from build123d import *

# Parameters (mm, degrees)
SKETCH1_R           = 25
BOSS_EXTRUDE1_DEPTH = 40
SKETCH2_R           = 60
BOSS_EXTRUDE2_DEPTH = 50
CHAMFER1_SIZE       = 7.5
CUT_EXTRUDE1_DEPTH  = 3


with BuildPart() as part:
    # Sketch1 → Boss-Extrude1 (new body)
    with BuildSketch(Plane(origin=(0, 0, 0), x_dir=(1, 0, 0), z_dir=(0, 1, 0))):
        with Locations(Location((0, 0, 0), (0, 0, 270))):
            Circle(SKETCH1_R)
    extrude(amount=BOSS_EXTRUDE1_DEPTH)

    # Sketch2 → Boss-Extrude2 (add)
    with BuildSketch(Plane(origin=(0, 40, 0), x_dir=(1, 0, 0), z_dir=(0, 1, 0))):
        with Locations(Location((0, 0, 0), (0, 0, 270))):
            Circle(SKETCH2_R)
    extrude(amount=BOSS_EXTRUDE2_DEPTH)

    # Chamfer1
    chamfer1_edges = [part.edges().sort_by_distance(p)[0] for p in [
        (0, 90, -60),
    ]]
    chamfer(chamfer1_edges, length=CHAMFER1_SIZE)

    # Sketch3 → Cut-Extrude1 (cut)
    with BuildSketch(Plane(origin=(0, 90, 0), x_dir=(1, 0, 0), z_dir=(0, 1, 0))):
        with BuildLine():
            Line((-3, 1.732050808), (-53.461524227, -27.401923789))
            ThreePointArc((-53.461524227, -27.401923789), (-54.559600438, -31.5), (-50.461524227, -32.598076211))
            Line((-50.461524227, -32.598076211), (0, -3.464101615))
            Line((0, -3.464101615), (50.461524227, -32.598076211))
            ThreePointArc((50.461524227, -32.598076211), (54.559600438, -31.5), (53.461524227, -27.401923789))
            Line((53.461524227, -27.401923789), (3, 1.732050808))
            Line((3, 1.732050808), (3, 60))
            ThreePointArc((3, 60), (0, 63), (-3, 60))
            Line((-3, 60), (-3, 1.732050808))
        make_face()
    extrude(amount=-CUT_EXTRUDE1_DEPTH, mode=Mode.SUBTRACT)


solid = part.part
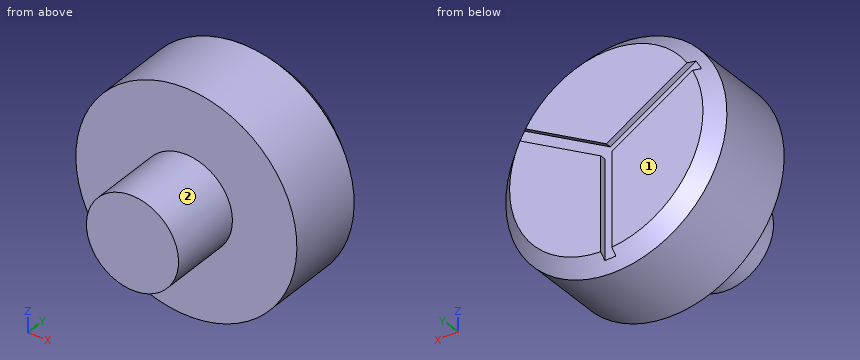
The model under review builds one solid part; all positions refer to its coordinate system, in mm. Face numbers are marked on the shaded views. A direction names the side the tool comes from. Coordinates: 2 decimals unless noted, no trailing zeros. Write each loop counter-clockwise with the first axis right and the second up, starting at its lowest first coordinate (ties: lowest second). Pieces come first, ordered by that corner, then holes. Notation, with made-up numbers: (39, 79) - (98, 79) arc R18 ccw to (98, 104) - close; hole circle Ø7 at (-3.5, -15). An arc over 180 degrees is marked (long way). Answer as CSV lines item,"result".
(1) We need section A-A (z = 0). Give the boundary of the cut face in (x, y), plus the area to 3 significant figures.
Data:
outline,"(-60, 40) - (-25, 40) - (-25, 0) - (25, 0) - (25, 40) - (60, 40) - (60, 82.5) - (52.5, 90) - (6, 90) - (6, 87) - (-6, 87) - (-6, 90) - (-52.5, 90) - (-60, 82.5) - close"
area,"7,910 mm2"
(2) We need section C-C (y = 8). Give the boundary of the cut face in (x, z), plus the area to 3 significant figures.
Data:
outline,"circle Ø50 at (0, 0)"
area,"1,960 mm2"
(3) Tool access review of the marked faces 1 and 2: name each direction out of +Z, -Z, +X, -X, +Y, -Y from which nothing blocks a thin tool from reaching the whole face with its end or side.
Data:
face 1,"+Z, -Z, +X, -X, +Y"
face 2,"-Y"
(4) We need section B-B (y = 80.5). Give the boundary of the cut face in (x, z).
Data:
outline,"circle Ø120 at (0, 0)"
(5) Clearance check with flat-ended pins moving along their axes: pin 1 Ø2 at (x, y) = (2.5, 14.5) entering from +Z; pin 2 Ø2 at (x, y) = (1.5, 57) entering from +Z; pin 3 Ø2 at (x, y) = (-12.5, 13.5) entering from -Z. State where each tip first meets the part, or that it passes through.
Data:
pin 1,"stops at z = 24.95"
pin 2,"stops at z = 60"
pin 3,"stops at z = -22.2"
(6) For line 1 along Y through (x, z) = (-15, 40); line 2 along Z through (x, y) = (0.5, 26.5) (3 decimals); line 3 along Y through (x, z) = (-5, 3), list the stretches that pass through material, from the lowest coordinate up. Write a range as [from, to].
Data:
line 1,"y = [40, 90]"
line 2,"z = [-24.995, 24.995]"
line 3,"y = [0, 87]"
